The model under review builds one solid part; all positions refer to its coordinate system, in mm. A direction names the side the tool comes from. Round coordinates to 2 decimals unless told otherwise and drop trailing zeros. Loops run counter-clockwise (first coordinate to the right, second up) from the corner with the lowest first, then second, coordinate; pieces in that order, holes last. Notation, with made-up numbers: M 12.5,-9 L 18.5,-9 A27 ccw 18.5,8 Z; hole C 9.25,75 d9. An arc over 180 degrees is marked long. Answer as a JSON object with one key per item and string values. Group by question number.
Item 1: Consider section D-D (y = 45). Give the boundary of the cut face in (x, z), and give its area (3 significant figures).
Item 2: Insertion check: P1, Ø8, axis at y = 9, z = 43, coming from the +X side; P2, Ø7.5, axis at y = 23, z = 92, coming from the -X side; P3, Ø3, axis at x = 46.5, z = 61, coming from the -Y side. Each pin has a flat end and moves straight along its axis. Give the tip position at first contact, or say it passes through.
Item 3: The part is to be moulded in two halves that separate along X. For faces 4 (the face through (0, 26, 4)), 5 (the face through (52.249, 25.151, 9.148)), 6 (the face through (47.71, 16.32, 135.88)), say which applies: +X half, -X half, draft (parallel to the pull), parting line (faces both ways), or undercut.
Item 4: To check wall thickness, follow line 1 (Y direction, x = 95, z = 4); line 2 (Y direction, x = 19.05, z = 3.5); line 3 (Z direction, x = 48, y = 25.4). State the ranges of each line that lie inside material, in increasing order.
Item 5: Consider section B-B (x = 95.25). Give the boundary of the cut face in (y, z), and give its area (3 significant figures).
Item 6: Consider section A-A (z = 64). Give the boundary of the cut face in (x, y).
Item 7: Consider section C-C (y = 10.16). Give the boundary of the cut face in (x, z).
Item 8: Tool access review of faces 1 (the face through (50.8, 26, 75)), 2 (the face through (48, 38.1, 69)), 3 (the face through (48, 12.7, 69)): name each direction out of +Z, -Z, +X, -X, +Y, -Y from which nothing blocks a thin tool from reaching the whole face with its end or side.
Autodesk Fusion 360 part; units mm, degrees
sketch "Sketch1" plane through (0, 0, 0) normal (0, 0, 1) x (1, 0, 0)
  line L0 (0, 0) -> (114.3, 0)
  line L1 (114.3, 0) -> (114.3, 50.8)
  line L2 (114.3, 50.8) -> (0, 50.8)
  line L3 (0, 50.8) -> (0, 0)
  point P0 (114.3, 25.4)
  point P1 (57.15, 0)
  dimension "d1" = 114.3
  dimension "d4" = 50.8
extrude "Extrude4" add sketch "Sketch1" along normal blind 7.62
sketch "Sketch2" plane through (0, 0, 7.62) normal (0, 0, 1) x (-1, 0, 0)
  line L0 (0, -50.8) -> (0, 0)
  line L1 (0, 0) -> (-114.3, 0)
  line L2 (-114.3, 0) -> (-114.3, -50.8)
  line L3 (-114.3, -50.8) -> (0, -50.8)
  line L4 (-44.704, -38.1) -> (-69.596, -38.1)
  line L5 (-69.596, -38.1) -> (-69.596, -12.7)
  line L6 (-69.596, -12.7) -> (-44.704, -12.7)
  line L7 (-44.704, -12.7) -> (-44.704, -38.1)
  line L8 (-63.5, -38.1) -> (-50.8, -38.1)
  line L9 (-50.8, -38.1) -> (-50.8, -12.7)
  line L10 (-50.8, -12.7) -> (-63.5, -12.7)
  line L11 (-63.5, -12.7) -> (-63.5, -38.1)
  line L12 (-63.5, -38.1) -> (-50.8, -12.7) construction
  line L13 (-50.8, -38.1) -> (-63.5, -12.7) construction
  circle A0 centre (-19.05, -40.64) radius 2.5
  line L14 (-57.15, -50.8) -> (-57.15, 0) construction
  line L15 (0, -25.4) -> (-114.3, -25.4) construction
  circle A1 centre (-95.25, -40.64) radius 2.5
  circle A2 centre (-19.05, -10.16) radius 2.5
  circle A3 centre (-95.25, -10.16) radius 2.5
  point P0 (-57.15, -38.1)
  point P1 (-69.596, -25.4)
  point P2 (-114.3, -25.4)
  point P3 (-57.15, 0)
  point P4 (-57.15, -25.4)
  dimension "d15" = 25.4
  dimension "d23" = 12.7
  dimension "d24" = 5
  dimension "d25" = 76.2
  dimension "d26" = 30.48
  dimension "d27" = 15.24
  dimension "d43" = 6.096
  dimension "d45" = 6.096
extrude "Extrude5" add sketch "Sketch2" along normal blind 132.08 contours L4 L6 L7 L9 | L4 L5 L6 L11
sketch "Sketch3" plane through (69.596, 0, 0) normal (1, 0, 0) x (0, 1, 0)
  line L0 (12.7, 7.62) -> (38.1, 7.62)
  line L1 (38.1, 7.62) -> (38.1, 139.7)
  line L2 (38.1, 139.7) -> (12.7, 139.7)
  line L3 (12.7, 139.7) -> (12.7, 7.62)
  circle A0 centre (25.4, 131.3981) radius 1.5
  circle A1 centre (25.4, 105.9981) radius 1.4986
  line L4 (25.4, 7.62) -> (25.4, 27.94) construction
  circle A2 centre (25.4, 80.5981) radius 1.4986
  circle A3 centre (25.4, 55.1981) radius 1.4986
  circle A4 centre (25.4, 29.7981) radius 1.4986
  point P0 (25.4, 139.7)
  dimension "d19" = 3
  dimension "d20" = 2.9972
  dimension "d21" = 25.4
  dimension "d37" = 2.9972
  dimension "d38" = 2.9972
  dimension "d39" = 2.9972
  dimension "d40" = 25.4
  dimension "d41" = 25.4
  dimension "d42" = 25.4
extrude "Extrude6" cut sketch "Sketch3" against normal through all contours A0 | A1 | A2 | A3 | A4
extrude "Extrude7" cut sketch "Sketch2" against normal through all contours A0 | A1 | A2 | A3
fillet "Fillet9" radius 12.7 4 edges at (66.548, 12.7, 139.7) (47.752, 12.7, 139.7) (47.752, 38.1, 139.7) (66.548, 38.1, 139.7)
fillet "Fillet10" radius 5.08 8 edges at (69.596, 25.4, 7.62) (66.548, 38.1, 7.62) (63.5, 25.4, 7.62) (44.704, 25.4, 7.62) (47.752, 38.1, 7.62) (50.8, 25.4, 7.62) (47.752, 12.7, 7.62) (66.548, 12.7, 7.62)
equation "d37 = d20"
equation "d38 = d20"
equation "d39 = d20"
equation "d45 = d43"
Geometry results:
{
 "1": {"outline": "M 0,0 L 114.3,0 L 114.3,7.62 L 0,7.62 Z", "area": "871 mm^2"},
 "2": {"P1": "stops at x = 69.6", "P2": "stops at x = 44.7", "P3": "stops at y = 12.7"},
 "3": {"face 4": "-X half", "face 5": "undercut", "face 6": "draft"},
 "4": {"line 1": "y = 0 to 7.67, 12.65 to 38.15, 43.13 to 50.8", "line 2": "y = 0 to 7.66, 12.66 to 38.14, 43.14 to 50.8", "line 3": "z = 0 to 28.3, 31.3 to 53.7, 56.7 to 79.1, 82.1 to 104.5, 107.5 to 129.9, 132.9 to 139.7"},
 "5": {"outline": "M 0,0 L 7.66,0 L 7.66,7.62 L 0,7.62 Z; M 12.66,0 L 38.14,0 L 38.14,7.62 L 12.66,7.62 Z; M 43.14,0 L 50.8,0 L 50.8,7.62 L 43.14,7.62 Z", "area": "311 mm^2"},
 "6": {"outline": "M 44.7,12.7 L 50.8,12.7 L 50.8,38.1 L 44.7,38.1 Z; M 63.5,12.7 L 69.6,12.7 L 69.6,38.1 L 63.5,38.1 Z"},
 "7": {"outline": "M 0,0 L 16.55,0 L 16.55,7.62 L 0,7.62 Z; M 21.55,0 L 92.75,0 L 92.75,7.62 L 74.68,7.62 A5.08 cw 72.14,8.3 L 60.96,8.3 A5.08 cw 58.42,7.62 L 55.88,7.62 A5.08 cw 53.34,8.3 L 42.16,8.3 A5.08 cw 39.62,7.62 L 21.55,7.62 Z; M 97.75,0 L 114.3,0 L 114.3,7.62 L 97.75,7.62 Z"},
 "8": {"face 1": "+Z, +Y, -Y", "face 2": "+Z, +X, -X, +Y", "face 3": "+Z, +X, -X, -Y"}
}
